from build123d import *

# Parameters (mm, degrees)
SKETCH1_W           = 29
SKETCH1_H           = 55.5
BODY_DEPTH          = 4
SKETCH2_R           = 1.5
BOLT_HOLES_DEPTH    = 63.747509911
CUT_EXTRUDE1_DEPTH  = 10
SKETCH6_W           = 25
SKETCH6_H           = 25
CUT_EXTRUDE2_DEPTH  = 2
SKETCH7_W           = 17
SKETCH7_H           = 2
BOSS_EXTRUDE1_DEPTH = 10.25
BOSS_EXTRUDE2_DEPTH = 17


with BuildPart() as part:
    # Sketch1 → Body (new body)
    with BuildSketch(Plane.XY):
        with Locations((14.5, 27.75)):
            Rectangle(SKETCH1_W, SKETCH1_H)
    extrude(amount=BODY_DEPTH)

    # Sketch2 → Bolt Holes (cut, through all)
    with BuildSketch(Plane.XY.offset(4)):
        with Locations((3, 52.385)):
            Circle(SKETCH2_R)
        with Locations(Location((26, 52.385, 0), (0, 0, 180))):
            Circle(SKETCH2_R)
        with Locations((26, 3.115)):
            Circle(SKETCH2_R)
        with Locations(Location((3, 3.115, 0), (0, 0, 180))):
            Circle(SKETCH2_R)
    extrude(amount=-BOLT_HOLES_DEPTH, mode=Mode.SUBTRACT)

    # Sketch4 → Cut-Extrude1 (cut)
    with BuildSketch(Plane.XY):
        with BuildLine():
            Line((4.563898139, 34.308305648), (4.563898139, 27.5))
            Line((4.563898139, 27.5), (24.563898139, 27.5))
            Line((24.563898139, 27.5), (24.563898139, 34.308305648))
            ThreePointArc((24.563898139, 34.308305648), (26.753898139, 37.718422948), (24.563898139, 41.128540248))
            Line((24.563898139, 41.128540248), (24.563898139, 47.5))
            Line((24.563898139, 47.5), (4.563898139, 47.5))
            Line((4.563898139, 47.5), (4.563898139, 41.128540248))
            ThreePointArc((4.563898139, 41.128540248), (2.373898139, 37.718422948), (4.563898139, 34.308305648))
        make_face()
    extrude(amount=CUT_EXTRUDE1_DEPTH, mode=Mode.SUBTRACT)

    # Sketch6 → Cut-Extrude2 (cut)
    with BuildSketch(Plane(origin=(0, 0, 0), x_dir=(-1, 0, 0), z_dir=(0, 0, -1))):
        with Locations((-14.5, 37)):
            Rectangle(SKETCH6_W, SKETCH6_H)
    extrude(amount=-CUT_EXTRUDE2_DEPTH, mode=Mode.SUBTRACT)

    # Sketch7 → Boss-Extrude1 (add)
    with BuildSketch(Plane.XY):
        with Locations((14.5, 23.5)):
            Rectangle(SKETCH7_W, SKETCH7_H)
    extrude(amount=-BOSS_EXTRUDE1_DEPTH)

    # Sketch8 → Boss-Extrude2 (add)
    with BuildSketch(Plane(origin=(23, 0, 0), x_dir=(0, 0, -1), z_dir=(1, 0, 0))):
        Polygon((10.25, 22.5), (10.25, 26.5), (11.25, 26.5), (13.25, 24.5), (13.25, 22.5), align=None)
    extrude(amount=-BOSS_EXTRUDE2_DEPTH)

    # SurfaceCut1
    split(bisect_by=Plane(origin=(0, 22.5, 0), x_dir=(-1, 0, 0), z_dir=(0, -1, 0)), keep=Keep.BOTTOM)


solid = part.part
Part model, mm, in its own coordinate system. A direction names the side the tool comes from. Coordinates: 2 decimals unless noted, no trailing zeros. Order: outer loops, then holes, each group sorted by start corner. A loop starts at its lowest first (then second) coordinate and runs counter-clockwise, first axis right, second up.
(1) Pull direction Y, two halves, no side cores. Call faces 5 (the face through (14.62, 25.51, -12.24)), 6 (the face through (27.19, 53.3, 2.03)), 7 (the face through (27, 37, 1)), 8 (the face through (14, 50, 0)): pulls with the +Y half, pulls with the -Y half, needs draft (parallel to the pull), parting line crosses it, or undercut.
Check sheet entries:
face 5: pulls with the +Y half
face 6: undercut
face 7: undercut
face 8: needs draft
(2) Tool access for faces 1 (the face through (16, 27, 2)), 2 (the face through (23, 24, -8)), 3 (the face through (15, 25, -10.25)), 4 (the face through (4.564, 31, 3)): list every direction of +Z, -Z, +X, -X, +Y, -Y with a clear straight run to the whole face (end or side of a thin tool).
Check sheet entries:
face 1: none
face 2: -Z, +X, +Y, -Y
face 3: +X, -X, +Y
face 4: +Z, -Z
(3) Slice it at C-C, the plane x = 26. Write the cut outline in (y, z) (3 decimals).
Check sheet entries:
outline: (22.5, 0) - (24.5, 0) - (24.5, 2) - (35.463, 2) - (35.463, 4) - (22.5, 4) - close; (39.974, 2) - (49.5, 2) - (49.5, 0) - (50.885, 0) - (50.885, 4) - (39.974, 4) - close; (53.885, 0) - (55.5, 0) - (55.5, 4) - (53.885, 4) - close
(4) Slice it at D-D, the plane z = -12. Write the cut outline in (x, y), and give its area (4 significant figures).
Check sheet entries:
outline: (6, 22.5) - (23, 22.5) - (23, 25.75) - (6, 25.75) - close
area: 55.25 mm2
(5) Probe L1, parallel to Y at x = 26, z = 1.3 (3 decimals); L2, parallel to X at y = 29, z = 3.25; L3, parallel to Y at x = 26, z = 2.45 (3 decimals). List the from-to ranges inside material, lowest first.
Check sheet entries:
L1: y = 22.5 to 24.5, 49.5 to 50.885, 53.885 to 55.5
L2: x = 0 to 4.56, 24.56 to 29
L3: y = 22.5 to 35.463, 39.974 to 50.885, 53.885 to 55.5
(6) Slice it at B-B, the plane x = 18.5. Write the cut outline in (y, z).
Check sheet entries:
outline: (22.5, -13.25) - (24.5, -13.25) - (26.5, -11.25) - (26.5, -10.25) - (24.5, -10.25) - (24.5, 2) - (27.5, 2) - (27.5, 4) - (22.5, 4) - close; (47.5, 2) - (49.5, 2) - (49.5, 0) - (55.5, 0) - (55.5, 4) - (47.5, 4) - close
(7) Pin check, flat tips, straight feed: pin 1 Ø2 at (y, z) = (44.5, 3) entering from -X; pin 2 Ø6 at (x, y) = (24, 49.5) entering from -Z; pin 3 Ø4.5 at (y, z) = (24, -9) entering from -X; pin 4 Ø6 at (x, z) = (11, -7) entering from +Y. Stop position of each tip, or through.
Check sheet entries:
pin 1: stops at x = 0
pin 2: stops at z = 0
pin 3: stops at x = 6
pin 4: stops at y = 24.5
(8) Slice it at A-A, the plane y = 47. Write the cut outline in (x, z).
Check sheet entries:
outline: (0, 0) - (2, 0) - (2, 2) - (4.56, 2) - (4.56, 4) - (0, 4) - close; (24.56, 2) - (27, 2) - (27, 0) - (29, 0) - (29, 4) - (24.56, 4) - close
